from build123d import *

# Parameters (mm, degrees)
SKETCH1_W           = 200
SKETCH1_H           = 100
BOSS_EXTRUDE1_DEPTH = 20
SKETCH2_R           = 3
CUT_EXTRUDE1_DEPTH  = 20
SKETCH3_R           = 6
CUT_EXTRUDE2_DEPTH  = 10


with BuildPart() as part:
    # Sketch1 → Boss-Extrude1 (new body)
    with BuildSketch(Plane(origin=(0, 0, 0), x_dir=(1, 0, 0), z_dir=(0, 1, 0))):
        Rectangle(SKETCH1_W, SKETCH1_H)
    extrude(amount=BOSS_EXTRUDE1_DEPTH)

    # Sketch2 → Cut-Extrude1 (cut)
    with BuildSketch(Plane(origin=(0, 20, 0), x_dir=(1, 0, 0), z_dir=(0, 1, 0))):
        with Locations((-25, 30.5)):
            Circle(SKETCH2_R)
        with Locations((25, -30.5)):
            Circle(SKETCH2_R)
        with Locations((-25, -30.5)):
            Circle(SKETCH2_R)
        with Locations((25, 30.5)):
            Circle(SKETCH2_R)
    extrude(amount=-CUT_EXTRUDE1_DEPTH, mode=Mode.SUBTRACT)

    # Sketch3 → Cut-Extrude2 (cut)
    with BuildSketch(Plane.XZ):
        with Locations((25, -30.5)):
            Circle(SKETCH3_R)
        with Locations((-25, -30.5)):
            Circle(SKETCH3_R)
        with Locations((25, 30.5)):
            Circle(SKETCH3_R)
        with Locations((-25, 30.5)):
            Circle(SKETCH3_R)
    extrude(amount=-CUT_EXTRUDE2_DEPTH, mode=Mode.SUBTRACT)


solid = part.part
Verification items for the finished model (mm, model axes). A direction names the side the tool comes from. Coordinates: 2 decimals unless noted, no trailing zeros. Loops run counter-clockwise (first coordinate to the right, second up) from the corner with the lowest first, then second, coordinate; pieces in that order, holes last. Notation, with made-up numbers: (-1.75, 86.5) -> (28.25, 86.5) arc R23 ccw to (28.25, 112.5) -> close; hole circle Ø11 at (11, 61.25). An arc over 180 degrees is marked (long way). Answer as a JSON object with one key per item and string values. Group by question number.
Item 1: Sectioned sample at A-A on x = -25. Record the boundary of the cut face in (y, z).
Item 2: Scan lines: probe 1 along Z at (x, y) = (-25, 16); probe 2 along X at (y, z) = (14, -30.5); probe 3 along Z at (x, y) = (25, 3). Record each from-to range of solid material in increasing order.
Item 3: Depth check by flat-ended pin: pin 1 (7 mm diameter, centred on x = 25, z = -30.5, fed in from +Y); pin 2 (7 mm diameter, centred on x = 25, z = -30.5, fed in from -Y). Enter the tip coordinate at first touch or a pass-through.
Item 4: Sectioned sample at B-B on z = -30.5. Record the boundary of the cut face in (x, y), plus the area to 3 significant figures.
Item 5: Tool access check on faces 5 (the cylindrical face through (23.699, 4.93, 24.643)), 6 (the cylindrical face through (-28, 15.1, 30.4)). Record the directions out of +Z, -Z, +X, -X, +Y, -Y that give a thin tool (end or side, any length) a straight path to the whole face; none if there is none.
Item 6: Mould release check, pull along Z, two halves, no side actions. Record for faces 1 (the flat face through (100, 10, 1)), 2 (the flat face through (-1, 10, 50)), 3 (the cylindrical face through (-26.301, 4.93, 24.643)), 4 (the cylindrical face through (22, 15.1, 30.4)): +Z half, -Z half, draft (parallel to the pull), parting line (faces both ways), or undercut.
Evaluation:
{
 "1": {"outline": "(0, -50) -> (20, -50) -> (20, -33.5) -> (10, -33.5) -> (10, -36.5) -> (0, -36.5) -> close; (0, -24.5) -> (10, -24.5) -> (10, -27.5) -> (20, -27.5) -> (20, 27.5) -> (10, 27.5) -> (10, 24.5) -> (0, 24.5) -> close; (0, 36.5) -> (10, 36.5) -> (10, 33.5) -> (20, 33.5) -> (20, 50) -> (0, 50) -> close"},
 "2": {"probe 1": "z = -50 to -33.5, -27.5 to 27.5, 33.5 to 50", "probe 2": "x = -100 to -28, -22 to 22, 28 to 100", "probe 3": "z = -50 to -36.5, -24.5 to 24.5, 36.5 to 50"},
 "3": {"pin 1": "stops at y = 20", "pin 2": "stops at y = 10"},
 "4": {"outline": "(-100, 0) -> (-31, 0) -> (-31, 10) -> (-28, 10) -> (-28, 20) -> (-100, 20) -> close; (-22, 10) -> (-19, 10) -> (-19, 0) -> (19, 0) -> (19, 10) -> (22, 10) -> (22, 20) -> (-22, 20) -> close; (28, 10) -> (31, 10) -> (31, 0) -> (100, 0) -> (100, 20) -> (28, 20) -> close", "area": "3,640 mm²"},
 "5": {"face 5": "-Y", "face 6": "+Y, -Y"},
 "6": {"face 1": "draft", "face 2": "+Z half", "face 3": "undercut", "face 4": "undercut"}
}
